Here's how the part is built. I have some questions about the finished solid (model axes, mm). Face numbers are marked on the shaded views. A direction names the side the tool comes from. Give positions to 0.01 mm unless a question says otherwise; leave off trailing zeros. Order: outer loops, then holes, each group sorted by start corner. A loop starts at its lowest first (then second) coordinate and runs counter-clockwise, first axis right, second up. Notation, with made-up numbers: M 19.5,4.5 L 35.5,4.5 A28 cw 35.5,41.5 Z; hole C -7.75,45.5 d5. An arc over 180 degrees is marked long. Use one line per item in the form item = value.
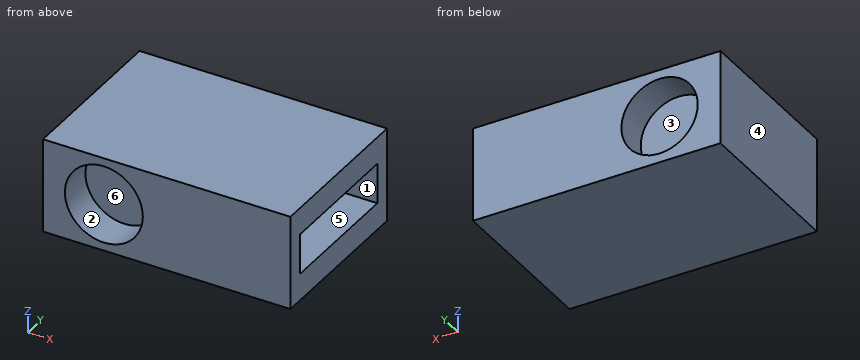
from build123d import *

# Parameters (mm, degrees)
F0_W     = 30
F0_H     = 20
F1_DEPTH = 5.715
F2_W     = 16
F2_H     = 4.89
F3_DEPTH = 15.24
F4_R     = 4.625
F5_DEPTH = 4
F6_R     = 4.725
F6_R_2   = 4.625
F7_DEPTH = 4.25


with BuildPart() as f1:
    # F0 (on Top) → F1 (new body, symmetric)
    with BuildSketch(Plane.XY):
        Rectangle(F0_W, F0_H)
    extrude(amount=F1_DEPTH, both=True)

    # F2 (on face) → F3 (cut)
    with BuildSketch(Plane.YZ.offset(15)):
        Rectangle(F2_W, F2_H)
    extrude(amount=-F3_DEPTH, mode=Mode.SUBTRACT)

    # F4 (on face) → F5 (cut)
    with BuildSketch(Plane(origin=(0, 10, 0), x_dir=(-1, 0, 0), z_dir=(0, 1, 0))):
        with Locations((7.62, 0)):
            Circle(F4_R)
    extrude(amount=-F5_DEPTH, mode=Mode.SUBTRACT)

    # F6 (on face) → F7 (cut)
    with BuildSketch(Plane.XZ.offset(10)):
        with Locations((-7.62, 0)):
            Circle(F6_R)
        with Locations((-7.62, 0)):
            Circle(F6_R_2, mode=Mode.SUBTRACT)
        with Locations((-7.62, 0)):
            Circle(F6_R_2)
    extrude(amount=-F7_DEPTH, mode=Mode.SUBTRACT)


solid = f1.part
Q1. I want a section at A-A on y = 6.75. Write out the boundary of the cut face in (x, z) (3 decimals).
Found:
outline = M -15,-5.715 L 15,-5.715 L 15,-2.445 L -0.24,-2.445 L -0.24,2.445 L 15,2.445 L 15,5.715 L -15,5.715 Z; hole C -7.62,0 d9.25
Q2. I want a section at C-C on z = 0. Write out the boundary of the cut face in (x, y) (3 decimals), then the cut area to 3 significant figures.
Found:
outline = M -15,-10 L -12.345,-10 L -12.345,-5.75 L -2.895,-5.75 L -2.895,-10 L 15,-10 L 15,-8 L -0.24,-8 L -0.24,8 L 15,8 L 15,10 L -2.995,10 L -2.995,6 L -12.245,6 L -12.245,10 L -15,10 Z
area = 279 mm²
Q3. I want a section at D-D on x = -7.62. Write out the boundary of the cut face in (y, z) (3 decimals), then the cut area to 3 significant figures.
Found:
outline = M -10,-5.715 L 10,-5.715 L 10,-4.625 L 6,-4.625 L 6,4.625 L 10,4.625 L 10,5.715 L -10,5.715 L -10,4.725 L -5.75,4.725 L -5.75,-4.725 L -10,-4.725 Z
area = 151 mm²
Q4. Thinking about a two-plate mould opening in X: for the marked faces 4, 5 and 6, which applies, +X half, -X half, draft (parallel to the pull), parting line (faces both ways), or undercut?
Found:
face_4 = -X half
face_5 = draft
face_6 = undercut
Q5. I'm going to push flat-ended pins straight in: pin 1 Ø2.5 at (y, z) = (0, 0.5) entering from +X; pin 2 Ø4.5 at (x, z) = (-8.5, 0.5) entering from +Y. Where does each tip first touch, or does it pass through?
Found:
pin_1 = -0.24
pin_2 = 6
Q6. I need wall thicknesses on L1, parallel to Z at x = 12, y = -7.75 (3 decimals); L2, parallel to Y at x = 7.25, z = -2; L3, parallel to Z at x = -7.62, y = -6.8 (3 decimals). Which ranges of each line are inside material? Lowest first, please.
Found:
L1 = -5.715 to -2.445, 2.445 to 5.715
L2 = -10 to -8, 8 to 10
L3 = -5.715 to -4.725, 4.725 to 5.715
Q7. I want a section at B-B on x = 6. Write out the boundary of the cut face in (y, z) (3 decimals), then the cut area to 3 significant figures.
Found:
outline = M -10,-5.715 L 10,-5.715 L 10,5.715 L -10,5.715 Z; hole M -8,-2.445 L 8,-2.445 L 8,2.445 L -8,2.445 Z
area = 150 mm²
Q8. On a 3-axis mill with a long thin cutter (end or side, diameter ignored), from which of +Z, -Z, +X, -X, +Y, -Y can I reach the whole of each face in a straight line? I mean the marked faces 1, 2 and 3. Say none if no direction works.
Found:
face_1 = +X
face_2 = -Y
face_3 = +Y
